Study the drawing (mm; zero at the part's minimum x, y, z) and answer. Round coordinates to 2 decimals unless told otherwise and drop trailing zeros. Write each loop counter-clockwise with the first axis right and the second up, starting at its lowest first coordinate (ties: lowest second). Pieces come first, ordered by that corner, then holes. Notation, with made-up numbers: M -11.5,28.25 L 40.5,28.25 A8 cw 40.5,38.25 Z; hole C 7.5,14 d11. An arc over 180 degrees is marked long. Write each question's results on one line, items separated by ' | '.
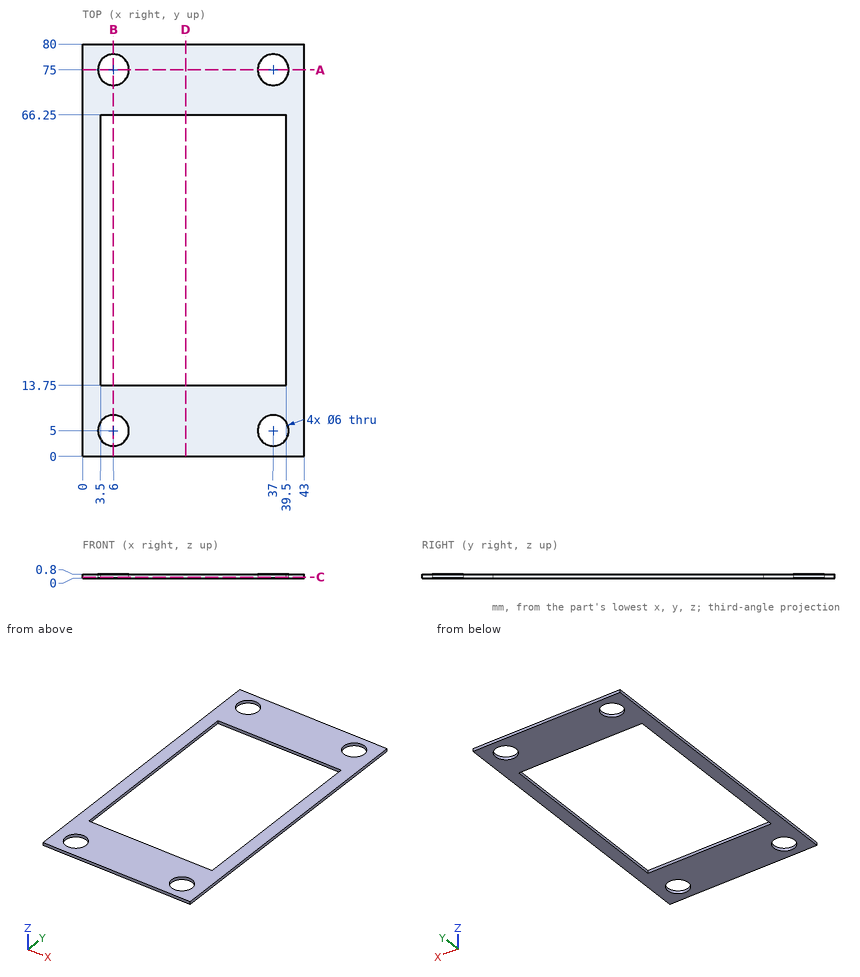
1) Section C-C (z = 0.25) is taken. Determine the outline of the cut face in (x, y), then the cut area to 3 significant figures.
Return value:
outline: M 0,0 L 43,0 L 43,80 L 0,80 Z; hole C 6,5 d6; hole C 6,75 d6; hole M 3.5,13.75 L 39.5,13.75 L 39.5,66.25 L 3.5,66.25 Z; hole C 37,5 d6; hole C 37,75 d6 | area: 1,440 mm²
2) Section D-D (x = 20) is taken. Determine the outline of the cut face in (y, z).
Return value:
outline: M 0,0 L 13.75,0 L 13.75,0.8 L 0,0.8 Z; M 66.25,0 L 80,0 L 80,0.8 L 66.25,0.8 Z
3) Find the intervals of material crossed by line 1 (Y direction, x = 6, z = 0.25); line 2 (X direction, y = 58.5, z = 0.65); line 3 (Y direction, x = 25, z = 0.5), in increasing order.
Return value:
line 1: 0 to 2, 8 to 13.75, 66.25 to 72, 78 to 80 | line 2: 0 to 3.5, 39.5 to 43 | line 3: 0 to 13.75, 66.25 to 80
4) Section B-B (x = 6) is taken. Determine the outline of the cut face in (y, z).
Return value:
outline: M 0,0 L 2,0 L 2,0.8 L 0,0.8 Z; M 8,0 L 13.75,0 L 13.75,0.8 L 8,0.8 Z; M 66.25,0 L 72,0 L 72,0.8 L 66.25,0.8 Z; M 78,0 L 80,0 L 80,0.8 L 78,0.8 Z
5) Section A-A (y = 75) is taken. Determine the outline of the cut face in (x, z), then the cut area to 3 significant figures.
Return value:
outline: M 0,0 L 3,0 L 3,0.8 L 0,0.8 Z; M 9,0 L 34,0 L 34,0.8 L 9,0.8 Z; M 40,0 L 43,0 L 43,0.8 L 40,0.8 Z | area: 24.8 mm²
